```python
from build123d import *

# Parameters (mm, degrees)
CROQUIS2_W              = 82
CROQUIS2_H              = 82
CORTAR_EXTRUIR1_DEPTH   = 11.5
SALIENTE_EXTRUIR1_DEPTH = 10.5
CROQUIS4_W              = 14
CROQUIS4_H              = 8.5
CORTAR_EXTRUIR2_DEPTH   = 10.5
CROQUIS5_R              = 1.5
CORTAR_EXTRUIR3_DEPTH   = 10


with BuildPart() as part:
    # Croquis1 → Revolución1 (revolve)
    with BuildSketch(Plane.XY):
        Polygon((-96.901642817, 61.97611702), (-96.901642817, 60.97611702), (-67.901642817, 60.97611702), (-67.901642817, 61.97611702), (-67.901642817, 71.97611702), (-86.901642817, 71.97611702), (-86.901642817, 61.97611702), align=None)
    revolve(axis=Axis((-26.901642817, 46.97611702, 0), (0, -1, 0)))

    # Croquis2 → Cortar-Extruir1 (cut)
    with BuildSketch(Plane(origin=(0, 71.97611702, 0), x_dir=(1, 0, 0), z_dir=(0, 1, 0))):
        with Locations((-26.901642817, 0)):
            Rectangle(CROQUIS2_W, CROQUIS2_H)
    extrude(amount=-CORTAR_EXTRUIR1_DEPTH, mode=Mode.SUBTRACT)

    # Croquis3 → Saliente-Extruir1 (add)
    with BuildSketch(Plane(origin=(0, 71.97611702, 0), x_dir=(1, 0, 0), z_dir=(0, 1, 0))):
        with BuildLine():
            Line((32.419516983, 9), (25.098357183, 9))
            Line((25.098357183, 9), (25.098357183, -9))
            Line((25.098357183, -9), (32.419516983, -9))
            ThreePointArc((32.419516983, -9), (33.098357183, 0), (32.419516983, 9))
        make_face()
    extrude(amount=SALIENTE_EXTRUIR1_DEPTH)

    # Croquis4 → Cortar-Extruir2 (cut)
    with BuildSketch(Plane.ZY.offset(-25.098357183)):
        with Locations((0, 77.22611702)):
            Rectangle(CROQUIS4_W, CROQUIS4_H)
    extrude(amount=-CORTAR_EXTRUIR2_DEPTH, mode=Mode.SUBTRACT)

    # Croquis5 → Cortar-Extruir3 (cut)
    with BuildSketch(Plane(origin=(0, 61.97611702, 0), x_dir=(1, 0, 0), z_dir=(0, 1, 0))):
        with Locations((-26.901642817, -65)):
            Circle(CROQUIS5_R)
        with Locations((-83.193294063, 32.5)):
            Circle(CROQUIS5_R)
        with Locations((29.390008429, 32.5)):
            Circle(CROQUIS5_R)
    extrude(amount=-CORTAR_EXTRUIR3_DEPTH, mode=Mode.SUBTRACT)


solid = part.part
```
Input: part model. Units: mm. Frame: model coordinates. A direction names the side the tool comes from. Round coordinates to 2 decimals unless told otherwise and drop trailing zeros. Write each loop counter-clockwise with the first axis right and the second up, starting at its lowest first coordinate (ties: lowest second). Pieces come first, ordered by that corner, then holes. Notation, with made-up numbers: (50.25, 11) - (81.25, 11) arc R6 ccw to (81.25, 18) - close; hole circle Ø8 at (7, -7). An arc over 180 degrees is marked (long way). Write item = value, one per line.
(1) Access query for faces 1 (the flat face through (-6, 61.976, 57)), 2 (the flat face through (29, 77, 7)), 3 (the flat face through (29, 77, 9)), 4 (the flat face through (14.098, 67, 1)). Directions: +Z, -Z, +X, -X, +Y, -Y. A direction counts if a zero-diameter tool reaches every point of the face in a straight line with its end or side. Return the directions, or none.
Geometry check:
face_1 = +Y
face_2 = +X, -X
face_3 = +Z, +X, -X, +Y
face_4 = +Y, -Y
(2) Section query D-D on y = 67.5. Output: boundary loops of the cut face in (x, z), then the cut area to 3 significant figures.
Geometry check:
outline = circle Ø120 at (-26.9, 0); hole (-67.9, -41) - (14.1, -41) - (14.1, 41) - (-67.9, 41) - close
area = 4,590 mm^2
(3) Material intervals for probe 1 along X at (y, z) = (61.6, -32.5); probe 2 along Y at (x, z) = (-17.5, 45); probe 3 along X at (y, z) = (70.75, -24.5), sorted ascending.
Geometry check:
probe_1 = -88.9 to -84.69, -81.69 to -67.9, 14.1 to 27.89, 30.89 to 35.1
probe_2 = 60.98 to 71.98
probe_3 = -81.67 to -67.9, 14.1 to 27.87
(4) Section query B-B on x = 11. Output: boundary loops of the cut face in (y, z).
Geometry check:
outline = (60.98, -58.85) - (61.98, -58.85) - (61.98, -46.51) - (71.98, -46.51) - (71.98, -41) - (60.98, -41) - close; (60.98, 41) - (71.98, 41) - (71.98, 46.51) - (61.98, 46.51) - (61.98, 58.85) - (60.98, 58.85) - close
(5) Pull-direction query (Z, two-part tool) for faces 5 (the cylindrical face through (28.65, 61.47, 42.59)), 6 (the flat face through (29, 77, -9)), 7 (the flat face through (29, 72.976, 0)), 8 (the flat face through (-27, 67, 41)); classes: +Z half, -Z half, draft (parallel to the pull), parting line (faces both ways), or undercut.
Geometry check:
face_5 = parting line
face_6 = -Z half
face_7 = undercut
face_8 = undercut
(6) Contact query for flat-ended pins moving along their axis: pin 1 Ø4 at (y, z) = (67, -50.5) entering from +X; pin 2 Ø8.5 at (x, y) = (29, 76.5) entering from -Z; pin 3 Ø11.5 at (y, z) = (77.5, -3.5) entering from -X; pin 4 Ø6 at (x, z) = (-76, 53) entering from -Y. Output: stop coordinate, or through.
Geometry check:
pin_1 = 8.42
pin_2 = -9
pin_3 = -86.87
pin_4 = 60.98
(7) Section query C-C on z = 22.5. Output: boundary loops of the cut face in (x, y).
Geometry check:
outline = (-93.19, 60.98) - (-67.9, 60.98) - (-67.9, 71.98) - (-82.52, 71.98) - (-82.52, 61.98) - (-93.19, 61.98) - close; (14.1, 60.98) - (39.38, 60.98) - (39.38, 61.98) - (28.72, 61.98) - (28.72, 71.98) - (14.1, 71.98) - close
(8) Section query A-A on z = 0. Output: boundary loops of the cut face in (x, y), then the cut area to 3 significant figures.
Geometry check:
outline = (-96.9, 60.98) - (-67.9, 60.98) - (-67.9, 71.98) - (-86.9, 71.98) - (-86.9, 61.98) - (-96.9, 61.98) - close; (14.1, 60.98) - (43.1, 60.98) - (43.1, 61.98) - (33.1, 61.98) - (33.1, 72.98) - (25.1, 72.98) - (25.1, 71.98) - (14.1, 71.98) - close; (25.1, 81.48) - (33.1, 81.48) - (33.1, 82.48) - (25.1, 82.48) - close
area = 454 mm^2
